Work out the finished part from the listing and answer in its coordinate system (mm). Face numbers are marked on the shaded views. A direction names the side the tool comes from. Round coordinates to 2 decimals unless told otherwise and drop trailing zeros. Loops run counter-clockwise (first coordinate to the right, second up) from the corner with the lowest first, then second, coordinate; pieces in that order, holes last. Notation, with made-up numbers: (81, 69.25) -> (127, 69.25) arc R31 ccw to (127, 94.25) -> close; hole circle Ø3 at (59.25, -6). An arc over 180 degrees is marked (long way). Write item = value, one per line. Start each with the question number.
```python
from build123d import *

# Parameters (mm, degrees)
BOX001_W     = 2
BOX001_H     = 44
BOX001_DEPTH = 44
BOX002_W     = 2
BOX002_H     = 44
BOX002_DEPTH = 44
BOX003_W     = 2
BOX003_H     = 44
BOX003_DEPTH = 44
BOX_W        = 2
BOX_H        = 44
BOX_DEPTH    = 44


with BuildPart() as cubo001:
    # Box001 → Box001 (new body)
    with BuildSketch(Plane(origin=(0, 0, 0), x_dir=(0, -1, 0), z_dir=(0, 0, 1))):
        with Locations((1, 22)):
            Rectangle(BOX001_W, BOX001_H)
    extrude(amount=BOX001_DEPTH)


with BuildPart() as cubo002:
    # Box002 → Box002 (new body)
    with BuildSketch(Plane(origin=(0, 46, 0), x_dir=(0, -1, 0), z_dir=(0, 0, 1))):
        with Locations((1, 22)):
            Rectangle(BOX002_W, BOX002_H)
    extrude(amount=BOX002_DEPTH)


with BuildPart() as cubo003:
    # Box003 → Box003 (new body)
    with BuildSketch(Plane(origin=(0, 0, 0), x_dir=(0, 0, -1), z_dir=(1, 0, 0))):
        with Locations((1, 22)):
            Rectangle(BOX003_W, BOX003_H)
    extrude(amount=BOX003_DEPTH)


with BuildPart() as fusion:
    # Box → Box (new body)
    with BuildSketch(Plane.XY):
        with Locations((1, 22)):
            Rectangle(BOX_W, BOX_H)
    extrude(amount=BOX_DEPTH)

    # Fusion: union Cubo001, Cubo002, Cubo003
    add(cubo001.part)
    add(cubo002.part)
    add(cubo003.part)


solid = fusion.part
```
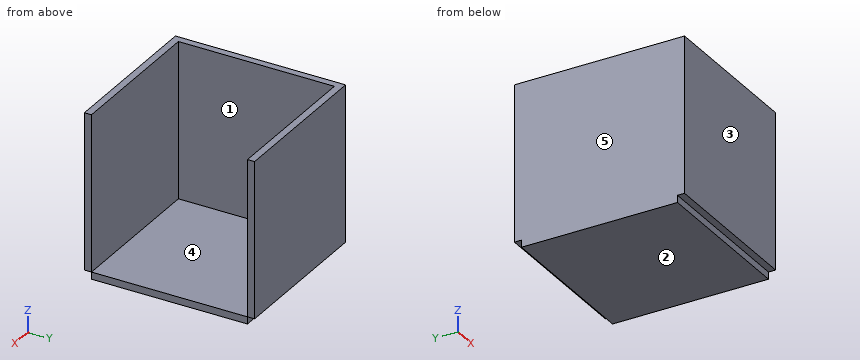
Item 1: Section B-B (z = 21) is taken. Determine the outline of the cut face in (x, y).
Item 2: Flat-ended cylindrical pins translate along their axes: pin 1 (1.6 mm diameter, centred on x = 27, z = -1, fed in from -Y); pin 2 (2 mm diameter, centred on y = 24, z = 9, fed in from -X); pin 3 (0.6 mm diameter, centred on x = 20, y = 45.5, fed in from -Z); pin 4 (1.5 mm diameter, centred on y = 20.5, z = 18, fed in from +X). Find the tip coordinate at first contact, or state that the pin passes through.
Item 3: The mould has two halves that part along Y. Classify the marked faces 1, 2 and 3: pulls with the +Y half, pulls with the -Y half, needs draft (parallel to the pull), parting line crosses it, or undercut.
Item 4: A tool of negligible diameter and unlimited length cuts with its end or side. For the marked faces 4 and 5, from which of +Z, -Z, +X, -X, +Y, -Y can it reach the whole face along a straight path? Write none if from no direction.
Item 5: Section C-C (y = 32) is taken. Determine the outline of the cut face in (x, z), then the cut area to 3 significant figures.
Item 6: Find the intervals of material crossed by line 1 along Y through (x, z) = (21.5, 37); line 2 along X through (y, z) = (32, 27.5); line 3 along Z through (x, y) = (11, 41), in increasing order. Write a range as [from, to].
Worked answers:
q1.outline = (0, -2) -> (44, -2) -> (44, 0) -> (2, 0) -> (2, 44) -> (44, 44) -> (44, 46) -> (0, 46) -> close
q2.pin_1 = 0
q2.pin_2 = 0
q2.pin_3 = 0
q2.pin_4 = 2
q3.face_1 = undercut
q3.face_2 = needs draft
q3.face_3 = pulls with the -Y half
q4.face_4 = +Z, +X
q4.face_5 = +Z, -Z, -X, +Y, -Y
q5.outline = (0, -2) -> (44, -2) -> (44, 0) -> (2, 0) -> (2, 44) -> (0, 44) -> close
q5.area = 176 mm2
q6.line_1 = [-2, 0], [44, 46]
q6.line_2 = [0, 2]
q6.line_3 = [-2, 0]
